```python
from build123d import *

# Parameters (mm, degrees)
BOSS_EXTRUDE1_DEPTH                      = 2.5
BOSS_EXTRUDE2_DEPTH                      = 0.5
F_2_5_2_5_DIAMETER_HOLE1_D               = 2.5
F_3_0_3_DIAMETER_HOLE1_D                 = 3
F_2_0_2_DIAMETER_HOLE1_D                 = 2
CBORE_FOR_M10_HEX_HEAD_BOLT1_D           = 11
CBORE_FOR_M10_HEX_HEAD_BOLT1_CBORE_D     = 12
CBORE_FOR_M10_HEX_HEAD_BOLT1_CBORE_DEPTH = 1


with BuildPart() as part:
    # Sketch1 → Boss-Extrude1 (new body)
    with BuildSketch(Plane.XY.offset(3)):
        with BuildLine():
            Line((-15, 0), (-15, -26))
            Line((-15, -26), (15, -26))
            Line((15, -26), (15, 0))
            ThreePointArc((15, 0), (0, 15), (-15, 0))
        make_face()
    extrude(amount=-BOSS_EXTRUDE1_DEPTH)

    # Sketch2 → Boss-Extrude2 (add)
    with BuildSketch(Plane(origin=(0, 0, 0.5), x_dir=(-1, 0, 0), z_dir=(0, 0, -1))):
        with BuildLine():
            Line((-14.25, -25.25), (-14.25, 0))
            ThreePointArc((-14.25, 0), (0, 14.25), (14.25, 0))
            Line((14.25, 0), (14.25, -25.25))
            Line((14.25, -25.25), (-14.25, -25.25))
        make_face()
    extrude(amount=BOSS_EXTRUDE2_DEPTH)

    # Ø2.5 (2.5) Diameter Hole1 (through all)
    with Locations(Plane(origin=(0, 0, 0), x_dir=(-1, 0, 0), z_dir=(0, 0, -1))):
        with Locations((9.25, -12.5), (-9.25, -12.5), (6.25, -16.5), (-6.25, -16.5)):
            Hole(F_2_5_2_5_DIAMETER_HOLE1_D / 2)

    # Ø3.0 (3) Diameter Hole1 (through all)
    with Locations(Plane(origin=(0, 0, 0), x_dir=(-1, 0, 0), z_dir=(0, 0, -1))):
        with Locations((-9.525, 0), (9.525, 0)):
            Hole(F_3_0_3_DIAMETER_HOLE1_D / 2)

    # Ø2.0 (2) Diameter Hole1 (through all)
    with Locations(Plane(origin=(0, 0, 0), x_dir=(-1, 0, 0), z_dir=(0, 0, -1))):
        with Locations((0, 10.45), (9.04996547, -5.225), (-9.04996547, -5.225)):
            Hole(F_2_0_2_DIAMETER_HOLE1_D / 2)

    # CBORE for M10 Hex Head Bolt1 (through all)
    with Locations(Plane.XY.offset(3)):
        with Locations((0, 0)):
            CounterBoreHole(CBORE_FOR_M10_HEX_HEAD_BOLT1_D / 2, CBORE_FOR_M10_HEX_HEAD_BOLT1_CBORE_D / 2, CBORE_FOR_M10_HEX_HEAD_BOLT1_CBORE_DEPTH)


solid = part.part
```
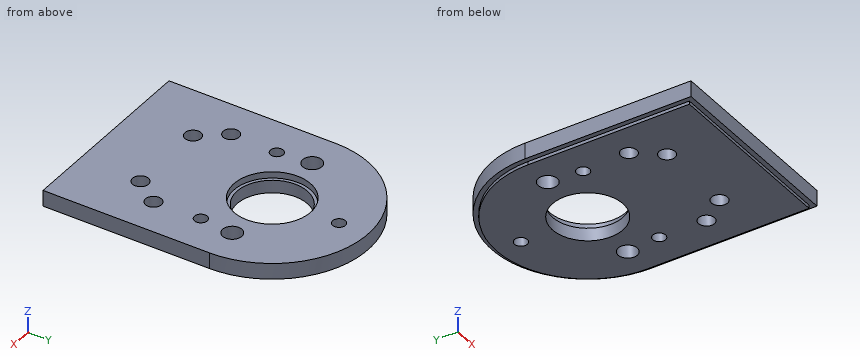
Read the model definition and answer for the solid it produces. Units are mm, in the model's axes. Coordinates: 2 decimals unless noted, no trailing zeros. Loops run counter-clockwise (first coordinate to the right, second up) from the corner with the lowest first, then second, coordinate; pieces in that order, holes last. Notation, with made-up numbers: (-11, 71.5) -> (22, 71.5) arc R21 ccw to (22, 78.5) -> close; hole circle Ø5 at (56.25, 70.25). An arc over 180 degrees is marked (long way). Return JSON: item names as keys, results as strings.
Item 1: Find the intervals of material crossed by probe 1 along Y at (x, z) = (0, 2.5); probe 2 along Y at (x, z) = (-0.5, 0.9); probe 3 along Y at (x, z) = (9.25, 0.95), in increasing order.
Answers:
{"probe 1": "y = -26 to -6, 6 to 9.45, 11.45 to 15", "probe 2": "y = -26 to -5.48, 5.48 to 9.58, 11.32 to 14.99", "probe 3": "y = -26 to -13.75, -11.25 to -6.2, -4.25 to -1.47, 1.47 to 11.81"}
Item 2: Find section A-A (y = -12.5). Determine the outline of the cut face in (x, z).
Answers:
{"outline": "(-15, 0.5) -> (-14.25, 0.5) -> (-14.25, 0) -> (-10.5, 0) -> (-10.5, 3) -> (-15, 3) -> close; (-8, 0) -> (8, 0) -> (8, 3) -> (-8, 3) -> close; (10.5, 0) -> (14.25, 0) -> (14.25, 0.5) -> (15, 0.5) -> (15, 3) -> (10.5, 3) -> close"}
Item 3: Find section C-C (x = 9.25). Determine the outline of the cut face in (y, z).
Answers:
{"outline": "(-26, 0.5) -> (-25.25, 0.5) -> (-25.25, 0) -> (-13.75, 0) -> (-13.75, 3) -> (-26, 3) -> close; (-11.25, 0) -> (-6.2, 0) -> (-6.2, 3) -> (-11.25, 3) -> close; (-4.25, 0) -> (-1.47, 0) -> (-1.47, 3) -> (-4.25, 3) -> close; (1.47, 0) -> (10.84, 0) -> (10.84, 0.5) -> (11.81, 0.5) -> (11.81, 3) -> (1.47, 3) -> close"}
Item 4: Find section B-B (x = -2.5). Determine the outline of the cut face in (y, z).
Answers:
{"outline": "(-26, 0.5) -> (-25.25, 0.5) -> (-25.25, 0) -> (-4.9, 0) -> (-4.9, 2) -> (-5.45, 2) -> (-5.45, 3) -> (-26, 3) -> close; (4.9, 0) -> (14.03, 0) -> (14.03, 0.5) -> (14.79, 0.5) -> (14.79, 3) -> (5.45, 3) -> (5.45, 2) -> (4.9, 2) -> close"}
Item 5: A flat-ended cylindrical pin translates along its axis: P1, Ø2, axis at x = -6.25, y = -16.5, coming from the -Z side. Find the tip coordinate at first contact, or state that the pin passes through.
Answers:
{"P1": "passes through"}
Item 6: Find section D-D (y = 10). Determine the outline of the cut face in (x, z).
Answers:
{"outline": "(-11.18, 0.5) -> (-10.15, 0.5) -> (-10.15, 0) -> (-0.89, 0) -> (-0.89, 3) -> (-11.18, 3) -> close; (0.89, 0) -> (10.15, 0) -> (10.15, 0.5) -> (11.18, 0.5) -> (11.18, 3) -> (0.89, 3) -> close"}
